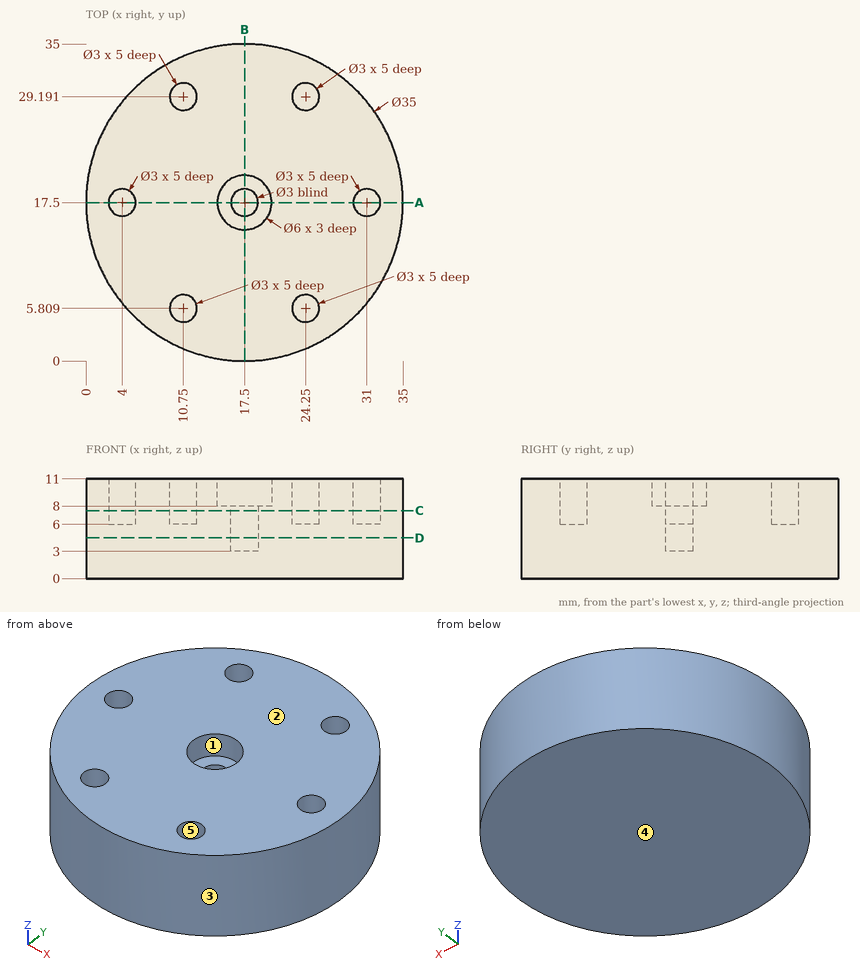
The drawing under review shows one solid part. Ordinate dimensions are in mm from its lowest x, y, z. A direction names the side the tool comes from. Coordinates: 2 decimals unless noted, no trailing zeros. Write each loop counter-clockwise with the first axis right and the second up, starting at its lowest first coordinate (ties: lowest second). Pieces come first, ordered by that corner, then holes. Notation, with made-up numbers: (52, -24.75) -> (63, -24.75) arc R20 cw to (63, 2.25) -> close; hole circle Ø3 at (0.25, 70). An arc over 180 degrees is marked (long way). One line per item, written item: value. Start each with the question number.
Q1. To check wall thickness, follow probe 1 along Y at (x, z) = (17.5, 9.15); probe 2 along Y at (x, z) = (24.25, 7.55) (1 decimal); probe 3 along X at (y, z) = (4.5, 10) (1 decimal). State the ranges of each line that lie inside material, in increasing order.
Q2. Clearance check with flat-ended pins moving along their axes: P1, Ø0.9, axis at x = 4, y = 17, coming from the +Z side; P2, Ø1.5, axis at x = 9, z = 10, coming from the -Y side; P3, Ø4, axis at x = 17.5, y = 17.5, coming from the +Z side. State where each tip first meets the part, or that it passes through.
Q3. The part is to be moulded in two halves that separate along Y. For the marked faces 3, 4 and 5, say which applies: +Y half, -Y half, draft (parallel to the pull), parting line (faces both ways), or undercut.
Q4. Add section C-C, the plane z = 7.5. Give the boundary of the cut face in (x, y), then the cut area to 3 significant figures.
Q5. Add section A-A, the plane y = 17.5. Give the boundary of the cut face in (x, z), then the cut area to 3 significant figures.
Q6. For the marked faces 1 and 2, list the 3-axis set-ups (+Z, -Z, +X, -X, +Y, -Y) from which the entire face can be reached by the end or side of a thin tool; tool diameter is ignored.
Q7. Add section B-B, the plane x = 17.5. Give the boundary of the cut face in (y, z).
Q8. Add section D-D, the plane z = 4.5. Give the boundary of the cut face in (x, y).
Response:
1. probe 1: 0 to 14.5, 20.5 to 35
1. probe 2: 1.4 to 4.3, 7.3 to 27.7, 30.7 to 33.6
1. probe 3: 5.8 to 10, 11.5 to 23.5, 25 to 29.2
2. P1: z = 6
2. P2: y = 1.81
2. P3: z = 8
3. face 3: parting line
3. face 4: draft
3. face 5: undercut
4. outline: circle Ø35 at (17.5, 17.5); hole circle Ø3 at (4, 17.5); hole circle Ø3 at (10.75, 5.81); hole circle Ø3 at (10.75, 29.19); hole circle Ø3 at (17.5, 17.5); hole circle Ø3 at (24.25, 5.81); hole circle Ø3 at (24.25, 29.19); hole circle Ø3 at (31, 17.5)
4. area: 913 mm²
5. outline: (0, 0) -> (35, 0) -> (35, 11) -> (32.5, 11) -> (32.5, 6) -> (29.5, 6) -> (29.5, 11) -> (20.5, 11) -> (20.5, 8) -> (19, 8) -> (19, 3) -> (16, 3) -> (16, 8) -> (14.5, 8) -> (14.5, 11) -> (5.5, 11) -> (5.5, 6) -> (2.5, 6) -> (2.5, 11) -> (0, 11) -> close
5. area: 322 mm²
6. face 1: +Z
6. face 2: +Z, +X, -X, +Y, -Y
7. outline: (0, 0) -> (35, 0) -> (35, 11) -> (20.5, 11) -> (20.5, 8) -> (19, 8) -> (19, 3) -> (16, 3) -> (16, 8) -> (14.5, 8) -> (14.5, 11) -> (0, 11) -> close
8. outline: circle Ø35 at (17.5, 17.5); hole circle Ø3 at (17.5, 17.5)
